Source: three-view drawing plus pictorial views. Frame: mm from the lowest corner of the part. A direction names the side the tool comes from. Give positions to 0.01 mm unless a question says otherwise; leave off trailing zeros. Order: outer loops, then holes, each group sorted by start corner. A loop starts at its lowest first (then second) coordinate and runs counter-clockwise, first axis right, second up. Notation, with made-up numbers: (3.5, 11.25) -> (58.5, 11.25) arc R24 cw to (58.5, 24.25) -> close; hole circle Ø3 at (31.5, -13.5). An arc over 180 degrees is marked (long way). Answer in a Markdown table with one row per item. Add a question column.
Q1. Contact query for flat-ended pins moving along their axis: P1, Ø1, axis at y = 56.5, z = 23, coming from the +X side; P2, Ø5.5, axis at y = 16, z = 28, coming from the +X side; P3, Ø10.5, axis at x = 128.61, y = 15.52, coming from the +Z side. Output: stop coordinate, or through.
Q2. Cut plane B-B on y = 37.5. Return the cut outline in (x, z) (1 decimal), and give its area (3 significant figures).
Q3. Cut plane A-A on y = 13.5. Return the cut outline in (x, z) (1 decimal).
Q4. Line query: line 1 along X through (y, z) = (18.5, 13) (1 decimal); line 2 along X through (y, z) = (45.5, 3.5) (1 decimal); line 3 along Z through (x, y) = (131, 52.5). Output: solid intervals per line, ascending. Write a range as from..to.
Q5. Cut plane C-C on z = 26.5. Return the cut outline in (x, y).
Q6. Cut plane D-D on y = 57.5. Return the cut outline in (x, z) (1 decimal), and give its area (3 significant figures).
Q7. Set-up query: the marked faces 1 and 2. Return all of +Z, -Z, +X, -X, +Y, -Y with unobstructed straight access to the full face (end or side cutting, diameter ignored); none if empty.
Q8. Pull-direction query (X, two-part tool) for the marked faces 3, 4 and 5; classes: +X half, -X half, draft (parallel to the pull), parting line (faces both ways), or undercut.
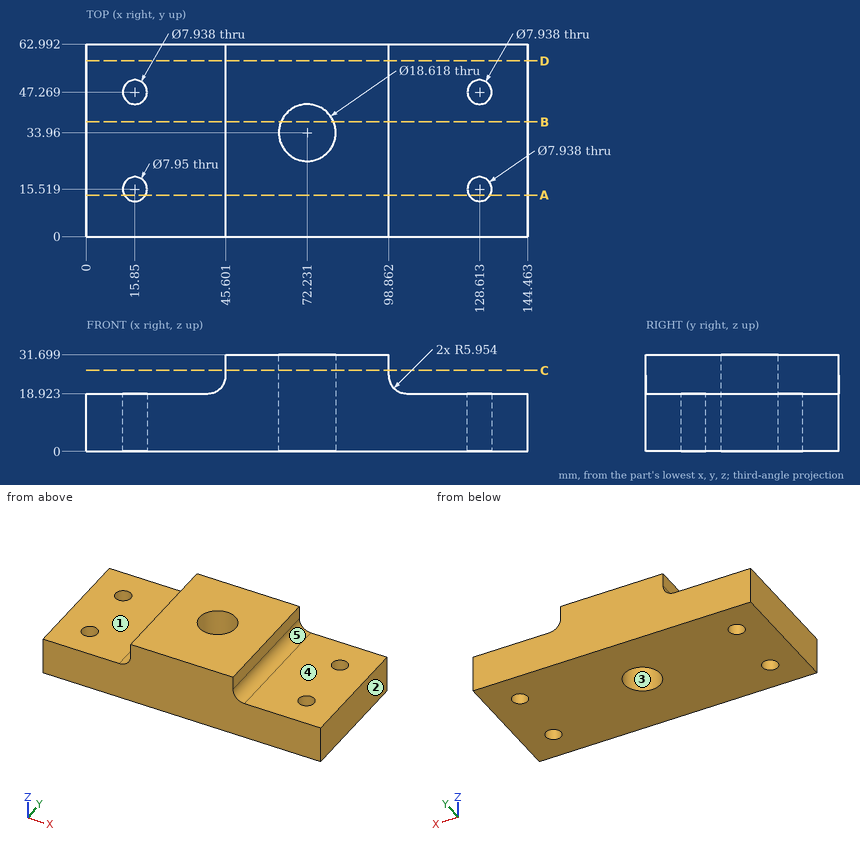
Completed:
| question | item | result |
|---|---|---|
| 1 | P1 | stops at x = 99.36 |
| 1 | P2 | stops at x = 98.86 |
| 1 | P3 | stops at z = 18.92 |
| 2 | outline | (0, 0) -> (63.6, 0) -> (63.6, 31.7) -> (45.6, 31.7) -> (45.6, 24.9) arc R6 cw to (39.6, 18.9) -> (0, 18.9) -> close; (80.8, 0) -> (144.5, 0) -> (144.5, 18.9) -> (104.8, 18.9) arc R6 cw to (98.9, 24.9) -> (98.9, 31.7) -> (80.8, 31.7) -> close |
| 2 | area | 2,880 mm² |
| 3 | outline | (0, 0) -> (12.4, 0) -> (12.4, 18.9) -> (0, 18.9) -> close; (19.3, 0) -> (125.2, 0) -> (125.2, 18.9) -> (104.8, 18.9) arc R6 cw to (98.9, 24.9) -> (98.9, 31.7) -> (45.6, 31.7) -> (45.6, 24.9) arc R6 cw to (39.6, 18.9) -> (19.3, 18.9) -> close; (132, 0) -> (144.5, 0) -> (144.5, 18.9) -> (132, 18.9) -> close |
| 4 | line 1 | x = 0..13.2, 18.5..126, 131.2..144.5 |
| 4 | line 2 | x = 0..12.3, 19.4..125.1, 132.2..144.5 |
| 4 | line 3 | z = 0..18.92 |
| 5 | outline | (45.6, 0) -> (98.86, 0) -> (98.86, 62.99) -> (45.6, 62.99) -> close; hole circle Ø18.62 at (72.23, 33.96) |
| 6 | outline | (0, 0) -> (144.5, 0) -> (144.5, 18.9) -> (104.8, 18.9) arc R6 cw to (98.9, 24.9) -> (98.9, 31.7) -> (45.6, 31.7) -> (45.6, 24.9) arc R6 cw to (39.6, 18.9) -> (0, 18.9) -> close |
| 6 | area | 3,430 mm² |
| 7 | face 1 | +Z, -X, +Y, -Y |
| 7 | face 2 | +Z, -Z, +X, +Y, -Y |
| 8 | face 3 | undercut |
| 8 | face 4 | draft |
| 8 | face 5 | +X half |
